```python
from build123d import *

# Parameters (mm, degrees)
SKETCH1_W                     = 30
SKETCH1_H                     = 180
BASE_FLANGE1_DEPTH            = 1.89738
EDGE_FLANGE1_STRIP_W          = 12.66952
EDGE_FLANGE1_STRIP_H          = 1.89738
EDGE_FLANGE1_STRIP_CUT_DEPTH  = 160
EDGE_FLANGE1_RELIEF_W         = 13.61821
EDGE_FLANGE1_RELIEF_H         = 0.94869
EDGE_FLANGE1_RELIEF_CUT_DEPTH = 1.89738
EDGE_FLANGE1_DEPTH            = 160
CUT_EXTRUDE1_DEPTH            = 10
CUT_EXTRUDE2_DEPTH            = 10


# Sheet-metal steps are written as plain solids
with BuildPart() as part:
    # Sketch1 → Base-Flange1 (new body)
    with BuildSketch(Plane.XY):
        with Locations((-15, -23.144555198)):
            Rectangle(SKETCH1_W, SKETCH1_H)
    extrude(amount=-BASE_FLANGE1_DEPTH)

    # Edge-Flange1 strip (across the edge) → Edge-Flange1 strip cut (cut)
    with BuildSketch(Plane(origin=(0, -103.144555198, 0), x_dir=(-1, 0, 0), z_dir=(0, 1, 0))):
        with Locations((-1.89738, -0.94869)):
            Rectangle(EDGE_FLANGE1_STRIP_W, EDGE_FLANGE1_STRIP_H)
    extrude(amount=EDGE_FLANGE1_STRIP_CUT_DEPTH, mode=Mode.SUBTRACT)

    # Edge-Flange1 relief (on the sheet) → Edge-Flange1 relief cut (cut)
    with BuildSketch(Plane(origin=(-4.43738, -103.144555198, 0), x_dir=(-1, 0, 0), z_dir=(0, 0, 1))):
        with Locations((-5.860415, 0.474345)):
            Rectangle(EDGE_FLANGE1_RELIEF_W, EDGE_FLANGE1_RELIEF_H)
        with Locations((-5.860415, -160.474345)):
            Rectangle(EDGE_FLANGE1_RELIEF_W, EDGE_FLANGE1_RELIEF_H)
    extrude(amount=-EDGE_FLANGE1_RELIEF_CUT_DEPTH, mode=Mode.SUBTRACT)

    # Edge-Flange1 section (across the edge) → Edge-Flange1 (add)
    with BuildSketch(Plane(origin=(0, -103.144555198, 0), x_dir=(-1, 0, 0), z_dir=(0, 1, 0))):
        with BuildLine():
            Line((0, 2.54), (0, 28.10262))
            Line((0, 28.10262), (1.89738, 28.10262))
            Line((1.89738, 28.10262), (1.89738, 2.54))
            ThreePointArc((1.89738, 2.54), (2.641328776, 0.743948776), (4.43738, 0))
            Line((4.43738, 0), (4.43738, -1.89738))
            ThreePointArc((4.43738, -1.89738), (1.299678511, -0.597701489), (0, 2.54))
        make_face()
    extrude(amount=EDGE_FLANGE1_DEPTH)

    # Sketch9 → Cut-Extrude1 (cut)
    with BuildSketch(Plane.ZY.offset(1.89738)):
        with BuildLine():
            Line((23.82131, 45.355444802), (6.82131, 45.355444802))
            ThreePointArc((6.82131, 45.355444802), (4.32131, 47.855444802), (6.82131, 50.355444802))
            Line((6.82131, 50.355444802), (23.82131, 50.355444802))
            ThreePointArc((23.82131, 50.355444802), (26.32131, 47.855444802), (23.82131, 45.355444802))
        make_face()
        with BuildLine():
            Line((6.82131, -91.644555198), (23.82131, -91.644555198))
            ThreePointArc((23.82131, -91.644555198), (26.32131, -94.144555198), (23.82131, -96.644555198))
            Line((23.82131, -96.644555198), (6.82131, -96.644555198))
            ThreePointArc((6.82131, -96.644555198), (4.32131, -94.144555198), (6.82131, -91.644555198))
        make_face()
    extrude(amount=-CUT_EXTRUDE1_DEPTH, mode=Mode.SUBTRACT)

    # Sketch11 → Cut-Extrude2 (cut)
    with BuildSketch(Plane(origin=(0, 0, -1.89738), x_dir=(-1, 0, 0), z_dir=(0, 0, -1))):
        with BuildLine():
            Line((16.708962543, -105.144555198), (16.708962543, -85.144555198))
            ThreePointArc((16.708962543, -85.144555198), (19.208962543, -82.644555198), (21.708962543, -85.144555198))
            Line((21.708962543, -85.144555198), (21.708962543, -105.144555198))
            ThreePointArc((21.708962543, -105.144555198), (19.208962543, -107.644555198), (16.708962543, -105.144555198))
        make_face()
        with BuildLine():
            Line((16.708962543, 38.855444802), (16.708962543, 58.855444802))
            ThreePointArc((16.708962543, 58.855444802), (19.208962543, 61.355444802), (21.708962543, 58.855444802))
            Line((21.708962543, 58.855444802), (21.708962543, 38.855444802))
            ThreePointArc((21.708962543, 38.855444802), (19.208962543, 36.355444802), (16.708962543, 38.855444802))
        make_face()
    extrude(amount=-CUT_EXTRUDE2_DEPTH, mode=Mode.SUBTRACT)


solid = part.part
```
Model file for the job. Use its own axes, mm. A direction names the side the tool comes from. Give positions to 0.01 mm unless a question says otherwise; leave off trailing zeros. Order: outer loops, then holes, each group sorted by start corner. A loop starts at its lowest first (then second) coordinate and runs counter-clockwise, first axis right, second up.
1) Wall check: probe 1 along X at (y, z) = (-99.5, 12.5); probe 2 along Z at (x, y) = (-2.25, -69.5). Give the ranges that are in metal, low to high.
2) Saw through at B-B, the plane y = -47.5. Write the cut outline in (x, z).
3) 3-axis set-ups, long thin cutter, end or side, ignore diameter. For faces 1 (the cylindrical face through (-1.3, -24.3, -0.6)), 2 (the flat face through (0, -24, 15)), 3 (the flat face through (-1.5, 56.855, 10)), 4 (the flat face through (-1.897, -24, 16)): which of +Z, -Z, +X, -X, +Y, -Y reach the whole face in a straight line?
4) Saw through at C-C, the plane x = -19.75. Write the cut outline in (y, z).
5) Mould opens along Y. For faces 5 (the flat face through (-1.5, -103.145, 10)), 6 (the flat face through (-15, -22, -1.897)) say: +Y half, -Y half, draft (parallel to the pull), parting line (faces both ways), or undercut.
6) Saw through at A-A, the plane z = 18.25. Write the cut outline in (x, y), then the cut area to 3 significant figures.
7) Pin check, flat tips, straight feed: pin 1 (6 mm diameter, centred on x = -23, y = -6.5, fed in from +Z); pin 2 (0.9 mm diameter, centred on x = -1, z = 13, fed in from -Y); pin 3 (5 mm diameter, centred on y = -16, z = 21.5, fed in from -X). Stop position of each tip, or through.
Computed:
1. probe 1: x = -1.9 to 0
1. probe 2: z = -1.32 to 1.25
2. outline: (-30, -1.9) - (-4.44, -1.9) arc R4.44 ccw to (0, 2.54) - (0, 28.1) - (-1.9, 28.1) - (-1.9, 2.54) arc R2.54 cw to (-4.44, 0) - (-30, 0) - close
3. face 1: -Z, +X
3. face 2: +Z, -Z, +X, +Y, -Y
3. face 3: +Z, -Z, +X
3. face 4: +Z, -X, +Y, -Y
4. outline: (-113.14, -1.9) - (-107.59, -1.9) - (-107.59, 0) - (-113.14, 0) - close; (-82.7, -1.9) - (36.41, -1.9) - (36.41, 0) - (-82.7, 0) - close; (61.3, -1.9) - (66.86, -1.9) - (66.86, 0) - (61.3, 0) - close
5. face 5: undercut
5. face 6: draft
6. outline: (-1.9, -103.14) - (0, -103.14) - (0, -96.64) - (-1.9, -96.64) - close; (-1.9, -91.64) - (0, -91.64) - (0, 45.36) - (-1.9, 45.36) - close; (-1.9, 50.36) - (0, 50.36) - (0, 56.86) - (-1.9, 56.86) - close
6. area: 285 mm2
7. pin 1: stops at z = 0
7. pin 2: stops at y = -103.14
7. pin 3: stops at x = -1.9
